from build123d import *

# Parameters (mm, degrees)
SKETCH1_W           = 152.4
SKETCH1_H           = 76.2
BOSS_EXTRUDE1_DEPTH = 81.28
CUT_EXTRUDE1_DEPTH  = 73.66
SKETCH4_W           = 177.8
SKETCH4_H           = 76.2
REVOLVE1_ANGLE      = 17.5
CUT_EXTRUDE2_DEPTH  = 136.575102434
SKETCH5_W           = 25.4
SKETCH5_H           = 76.2
CUT_EXTRUDE3_DEPTH  = 45.72
FILLET1_R           = 7.62
FILLET2_R           = 25.4
SKETCH7_W           = 21.387890157
SKETCH7_H           = 5.413955727
CUT_EXTRUDE5_DEPTH  = 149.031271926
SKETCH8_W           = 2.486098051
SKETCH8_H           = 76.2
CUT_EXTRUDE6_DEPTH  = 119.538217147
SKETCH9_W           = 18.783789955
SKETCH9_H           = 17.145
CUT_EXTRUDE7_DEPTH  = 3.175


with BuildPart() as part:
    # Sketch1 → Boss-Extrude1 (new body)
    with BuildSketch(Plane(origin=(0, 0, 0), x_dir=(1, 0, 0), z_dir=(0, 1, 0))):
        Rectangle(SKETCH1_W, SKETCH1_H)
    extrude(amount=BOSS_EXTRUDE1_DEPTH)

    # Sketch2 → Cut-Extrude1 (cut)
    with BuildSketch(Plane(origin=(0, 81.28, 0), x_dir=(1, 0, 0), z_dir=(0, 1, 0))):
        Polygon((-76.2, 0), (-76.2, 5.08), (-43.18, 5.08), (62.978326754, 28.614734436), (76.2, 28.614734436), (76.2, 17.184734436), (62.978326754, 16.907219588), (-13.285212414, 0), (62.978326754, -16.907219588), (76.2, -17.184734436), (76.2, -28.614734436), (62.978326754, -28.614734436), (-43.18, -5.08), (-76.2, -5.08), align=None)
    extrude(amount=-CUT_EXTRUDE1_DEPTH, mode=Mode.SUBTRACT)

    # Sketch4 → Revolve1 (revolve)
    with BuildSketch(Plane(origin=(0, 7.62, 0), x_dir=(-1, 0, 0), z_dir=(0, -1, 0))):
        with Locations((-12.7, 0)):
            Rectangle(SKETCH4_W, SKETCH4_H)
    revolve(axis=Axis((-76.2, 7.62, 38.1), (0, 0, 1)), revolution_arc=REVOLVE1_ANGLE)

    # Sketch3 → Cut-Extrude2 (cut, through all)
    with BuildSketch(Plane(origin=(0, 81.28, 0), x_dir=(1, 0, 0), z_dir=(0, 1, 0))):
        Polygon((62.978326754, 38.1), (-76.2, 38.1), (-76.2, 11.43), (-43.18, 11.43), align=None)
        Polygon((-76.2, -11.43), (-43.18, -11.43), (62.978326754, -38.1), (-76.2, -38.1), align=None)
    extrude(amount=-CUT_EXTRUDE2_DEPTH, mode=Mode.SUBTRACT)

    # Sketch5 → Cut-Extrude3 (cut)
    with BuildSketch(Plane(origin=(0, 0, 0), x_dir=(-1, 0, 0), z_dir=(0, -1, 0))):
        with Locations((-88.9, 0)):
            Rectangle(SKETCH5_W, SKETCH5_H)
    extrude(amount=-CUT_EXTRUDE3_DEPTH, mode=Mode.SUBTRACT)

    # Fillet1
    fillet1_edges = [part.edges().sort_by_distance(p)[0] for p in [
        (-43.18, 49.655583004, 5.08),
        (-43.18, 49.655583004, -5.08),
    ]]
    fillet(fillet1_edges, radius=FILLET1_R)

    # Fillet2
    fillet2_edges = [part.edges().sort_by_distance(p)[0] for p in [
        (62.978326754, 66.391378932, 16.907219588),
        (62.978326754, 66.391378932, -16.907219588),
    ]]
    fillet(fillet2_edges, radius=FILLET2_R)

    # Sketch7 → Cut-Extrude5 (cut, through all)
    with BuildSketch(Plane.XY.offset(38.1)):
        with Locations((86.893945078, 58.378513289)):
            Rectangle(SKETCH7_W, SKETCH7_H)
    extrude(amount=-CUT_EXTRUDE5_DEPTH, mode=Mode.SUBTRACT)

    # Sketch8 → Cut-Extrude6 (cut, through all)
    with BuildSketch(Plane(origin=(0, 55.671535425, 0), x_dir=(1, 0, 0), z_dir=(0, 1, 0))):
        with Locations((96.226838981, 0)):
            Rectangle(SKETCH8_W, SKETCH8_H)
    extrude(amount=-CUT_EXTRUDE6_DEPTH, mode=Mode.SUBTRACT)

    # Sketch9 → Cut-Extrude7 (cut)
    with BuildSketch(Plane(origin=(0, 55.671535425, 0), x_dir=(1, 0, 0), z_dir=(0, 1, 0))):
        with Locations((85.591894978, 22.899734436)):
            Rectangle(SKETCH9_W, SKETCH9_H)
        with Locations((85.591894978, -22.899734436)):
            Rectangle(SKETCH9_W, SKETCH9_H)
    extrude(amount=-CUT_EXTRUDE7_DEPTH, mode=Mode.SUBTRACT)


solid = part.part
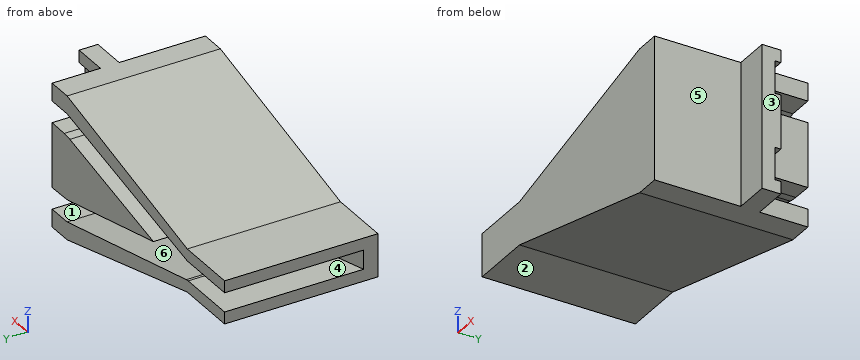
Input: part model. Units: mm. Frame: model coordinates. Face numbers are marked on the shaded views. A direction names the side the tool comes from. Round coordinates to 2 decimals unless told otherwise and drop trailing zeros. Write each loop counter-clockwise with the first axis right and the second up, starting at its lowest first coordinate (ties: lowest second). Pieces come first, ordered by that corner, then holes.
1) Cut plane D-D (y = 5.5). Return the cut outline in (x, z), then the cut area to 3 significant figures.
2) Cut plane A-A (y = 60). Return the cut outline in (x, z).
3) Reachability of the marked faces 4, 5 and 6 from +Z, -Z, +X, -X, +Y, -Y: full face, straight path, thin tool, end or side. Return the list, or none.
4) Contact query for flat-ended pins moving along their axis: P1, Ø8, axis at x = 58.5, y = 12.5, coming from the -Z side; P2, Ø1, axis at x = 20, y = 33.5, coming from the -Z side; P3, Ø10, axis at y = 59, z = 25, coming from the +X side. Output: stop coordinate, or through.
5) Cut plane B-B (z = 33.5). Return the cut outline in (x, y), then the cut area to 3 significant figures.
6) Ray query, L1, parallel to Z at x = 33, y = 44.5; L2, parallel to Z at x = -60.5, y = 29; L3, parallel to Z at x = 30, y = 75. Return the intervals inside material, ascending.
7) Cut plane C-C (x = 73.5). Return the cut outline in (y, z).
8) Draft query along Z for the marked faces 1, 2 and 3. Return one class per face: pulls with the +Z half, pulls with the -Z half, needs draft (parallel to the pull), parting line crosses it, or undercut.
Geometry says:
1. outline: (-76.2, -11.43) - (-43.18, -11.43) - (62.98, -38.1) - (76.2, -38.1) - (76.2, 38.1) - (62.98, 38.1) - (-43.18, 11.43) - (-76.2, 11.43) - close
1. area: 7,020 mm2
2. outline: (-76.2, -11.43) - (-43.18, -11.43) - (62.98, -38.1) - (76.2, -38.1) - (76.2, -28.61) - (62.98, -28.61) - (-42.37, -5.26) arc R7.62 ccw to (-44.01, -5.08) - (-76.2, -5.08) - close; (-76.2, 5.08) - (-44.01, 5.08) arc R7.62 ccw to (-42.37, 5.26) - (62.98, 28.61) - (76.2, 28.61) - (76.2, 38.1) - (62.98, 38.1) - (-43.18, 11.43) - (-76.2, 11.43) - close; (-13.29, 0) - (60.53, -16.36) arc R25.4 ccw to (65.49, -16.96) - (76.2, -17.18) - (76.2, 17.18) - (65.49, 16.96) arc R25.4 ccw to (60.53, 16.36) - close
3. face 4: -X, +Y
3. face 5: +Z, -Z, +X, -Y
3. face 6: +Y
4. P1: stops at z = -37.98
4. P2: stops at z = -27.43
4. P3: stops at x = 76.2
5. outline: (44.67, 0) - (76.2, 0) - (76.2, 45.72) - (94.98, 45.72) - (94.98, 55.67) - (76.2, 55.67) - (76.2, 81.28) - (44.67, 81.28) - close
5. area: 2,750 mm2
6. L1: z = -30.57 to -21.97, -10.26 to 10.26, 21.97 to 30.57
6. L2: z = -11.43 to -5.08, 5.08 to 11.43
6. L3: z = -29.81 to -21.3, -9.6 to 9.6, 21.3 to 29.81
7. outline: (0, -38.1) - (81.28, -38.1) - (81.28, -28.61) - (54.82, -28.61) - (54.82, -17.13) - (81.28, -17.13) - (81.28, 17.13) - (54.82, 17.13) - (54.82, 28.61) - (81.28, 28.61) - (81.28, 38.1) - (0, 38.1) - close
8. face 1: undercut
8. face 2: pulls with the -Z half
8. face 3: needs draft
